Part model, mm, in its own coordinate system. Face numbers are marked on the shaded views. Give positions to 0.01 mm unless a question says otherwise; leave off trailing zeros. Order: outer loops, then holes, each group sorted by start corner. A loop starts at its lowest first (then second) coordinate and runs counter-clockwise, first axis right, second up.
1. Mould opens along Y. For the marked faces 1, 2 and 3 say: +Y half, -Y half, draft (parallel to the pull), parting line (faces both ways), or undercut.
2. Slice it at D-D on y = 7.5. List the corners of the cut face in (x, z), and give its area (3 significant figures).
3. Slice it at B-B on x = 0. List the corners of the cut face in (y, z), and give its area (3 significant figures).
4. Probe line 1 (Y direction, x = 0, z = 5); line 2 (X direction, y = -16, z = 3.25); line 3 (Y direction, x = -17, z = 2.75). List the from-to ranges inside material, lowest first.
5. Drop flat-ended pins along their axis: pin 1 Ø6 at (x, y) = (0, 0) entering from -Z; pin 2 Ø2.5 at (x, y) = (0, 20) entering from -Z; pin 3 Ø2 at (x, z) = (7, 2.5) entering from +Y; pin 4 Ø3 at (x, z) = (16, 4.5) entering from -Y. Give the stop position or say it passes through.
6. Slice it at A-A on y = -15. List the corners of the cut face in (x, z), and give its area (3 significant figures).
7. Slice it at C-C on z = 3.5. Give the number of separate pieces and of enclosed holes in the cut face, and give its area (3 significant figures).
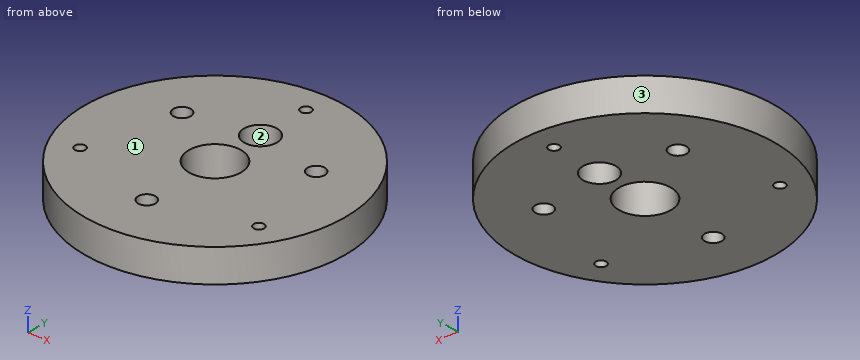
from build123d import *

# Parameters (mm, degrees)
SKETCH1_R           = 25
SKETCH1_R_2         = 5
SKETCH1_R_3         = 1
SKETCH1_R_4         = 3.15
SKETCH1_R_5         = 1.65
BOSS_EXTRUDE1_DEPTH = 6.3


with BuildPart() as part:
    # Sketch1 → Boss-Extrude1 (new body)
    with BuildSketch(Plane.XY):
        Circle(SKETCH1_R)
        Circle(SKETCH1_R_2, mode=Mode.SUBTRACT)
        with Locations((0, 20)):
            Circle(SKETCH1_R_3, mode=Mode.SUBTRACT)
        with Locations((17.320508076, -10)):
            Circle(SKETCH1_R_3, mode=Mode.SUBTRACT)
        with Locations((-17.320508076, -10)):
            Circle(SKETCH1_R_3, mode=Mode.SUBTRACT)
        with Locations((0, 10)):
            Circle(SKETCH1_R_4, mode=Mode.SUBTRACT)
        with Locations((-12.990381057, 7.5)):
            Circle(SKETCH1_R_5, mode=Mode.SUBTRACT)
        with Locations((12.990381057, 7.5)):
            Circle(SKETCH1_R_5, mode=Mode.SUBTRACT)
        with Locations((0, -15)):
            Circle(SKETCH1_R_5, mode=Mode.SUBTRACT)
    extrude(amount=BOSS_EXTRUDE1_DEPTH)


solid = part.part
Data:
1. face 1: draft
1. face 2: undercut
1. face 3: parting line
2. outline: (-23.85, 0) - (-14.64, 0) - (-14.64, 6.3) - (-23.85, 6.3) - close; (-11.34, 0) - (-1.92, 0) - (-1.92, 6.3) - (-11.34, 6.3) - close; (1.92, 0) - (11.34, 0) - (11.34, 6.3) - (1.92, 6.3) - close; (14.64, 0) - (23.85, 0) - (23.85, 6.3) - (14.64, 6.3) - close
2. area: 235 mm2
3. outline: (-25, 0) - (-16.65, 0) - (-16.65, 6.3) - (-25, 6.3) - close; (-13.35, 0) - (-5, 0) - (-5, 6.3) - (-13.35, 6.3) - close; (5, 0) - (6.85, 0) - (6.85, 6.3) - (5, 6.3) - close; (13.15, 0) - (19, 0) - (19, 6.3) - (13.15, 6.3) - close; (21, 0) - (25, 0) - (25, 6.3) - (21, 6.3) - close
3. area: 179 mm2
4. line 1: y = -25 to -16.65, -13.35 to -5, 5 to 6.85, 13.15 to 19, 21 to 25
4. line 2: x = -19.21 to -1.31, 1.31 to 19.21
4. line 3: y = -18.33 to -10.95, -9.05 to 18.33
5. pin 1: passes through
5. pin 2: stops at z = 0
5. pin 3: stops at y = 24.27
5. pin 4: stops at y = -20.37
6. outline: (-20, 0) - (-1.65, 0) - (-1.65, 6.3) - (-20, 6.3) - close; (1.65, 0) - (20, 0) - (20, 6.3) - (1.65, 6.3) - close
6. area: 231 mm2
7. separate pieces: 1
7. enclosed holes: 8
7. area: 1,820 mm2
